from build123d import *

# Parameters (mm, degrees)
SKETCH1_W           = 3
SKETCH1_H           = 7
BOSS_EXTRUDE1_DEPTH = 3


with BuildPart() as part:
    # Sketch1 → Boss-Extrude1 (new body)
    with BuildSketch(Plane(origin=(0, 0, 0), x_dir=(0, 0, -1), z_dir=(1, 0, 0))):
        Polygon((0, 50), (-10, 50), (-10, 0), (137.373870973, 0), (137.373870973, 3.192533317), (8.7714132, 50), align=None)
        Polygon((10.422986638, 46.206343112), (9.396926208, 43.387265249), (21.612930278, 38.941003386), (22.638990708, 41.760081248), align=None, mode=Mode.SUBTRACT)
        Polygon((34.854994778, 37.313819385), (33.828934348, 34.494741523), (46.044938419, 30.04847966), (47.070998848, 32.867557522), align=None, mode=Mode.SUBTRACT)
        Polygon((119.34096284, 3.37090848), (120.36702327, 6.189986343), (108.1510192, 10.636248206), (107.12495877, 7.817170343), align=None, mode=Mode.SUBTRACT)
        Polygon((95.935015129, 15.082510069), (94.908954699, 12.263432207), (82.692950629, 16.70969407), (83.719011059, 19.528771932), align=None, mode=Mode.SUBTRACT)
        Polygon((59.287002919, 28.421295659), (58.260942489, 25.602217796), (70.476946559, 21.155955933), (71.503006989, 23.975033796), align=None, mode=Mode.SUBTRACT)
        with Locations((-5.5, 38.5)):
            Rectangle(SKETCH1_W, SKETCH1_H, mode=Mode.SUBTRACT)
        with Locations((-5.5, 24.5)):
            Rectangle(SKETCH1_W, SKETCH1_H, mode=Mode.SUBTRACT)
        with Locations((-5.5, 10.5)):
            Rectangle(SKETCH1_W, SKETCH1_H, mode=Mode.SUBTRACT)
    extrude(amount=BOSS_EXTRUDE1_DEPTH)


solid = part.part
Can you work these out from the model? Positions are in its coordinate system, mm. A direction names the side the tool comes from. Coordinates: 2 decimals unless noted, no trailing zeros. Order: outer loops, then holes, each group sorted by start corner. A loop starts at its lowest first (then second) coordinate and runs counter-clockwise, first axis right, second up. Notation, with made-up numbers: (81, 77.25) - (108, 77.25) arc R34 cw to (108, 113.25) - close; hole circle Ø7 at (-31.5, 89). An arc over 180 degrees is marked (long way). Answer as a JSON object with one key per item and string values. Group by question number.
Q1. Imagine slicing it at C-C (x = 1.6). Give the number of separate pieces and of enclosed holes in the cut face, and give its area (3 significant figures).
Q2. We'd pull the mould along Z, two halves only. Please class faces 3 (the face through (1.479, 9.246, -107.645)), 4 (the face through (1, 2, -137.374)), 5 (the face through (1, 25, 10)), 6 (the face through (0, 20, -30)): +Z half, -Z half, draft (parallel to the pull), parting line (faces both ways), or undercut.
Q3. Will this pin go through, and if not, where does the flat tip stop? P1, Ø1.5, axis at y = 19.5, z = -79.5, coming from the -X side.
Q4. Imagine slicing it at A-A (z = -61.5). Please give me the cut outline in (x, y).
Q5. I need wall thicknesses on line 1 (Y direction, x = 0.6, z = -114.5); line 2 (Y direction, x = 0.7, z = -21); line 3 (Y direction, x = 2.8, z = -57.5). Which ranges of each line are inside material? Lowest first, please. Write a range as from..to.
Q6. Imagine slicing it at D-D (z = -115). Please give me the cut outline in (x, y).
Q7. On a 3-axis mill with a long thin cutter (end or side, diameter ignored), from which of +Z, -Z, +X, -X, +Y, -Y can I reach the whole of each face in a straight line? I mean faces 1 (the face through (1, 21, 6)), 2 (the face through (1.48, 26.27, -73.97)). Say none if no direction works.
Q8. Imagine slicing it at B-B (y = 40.5). Please give me the cut outline in (x, z), and give its area (3 significant figures).
Determined:
{
 "1": {"separate pieces": "1", "enclosed holes": "8", "area": "4,100 mm2"},
 "2": {"face 3": "undercut", "face 4": "-Z half", "face 5": "+Z half", "face 6": "draft"},
 "3": {"P1": "stops at x = 0"},
 "4": {"outline": "(0, 0) - (3, 0) - (3, 24.42) - (0, 24.42) - close; (0, 27.62) - (3, 27.62) - (3, 30.81) - (0, 30.81) - close"},
 "5": {"line 1": "y = 0..5.13, 8.33..11.52", "line 2": "y = 0..39.16, 42.36..45.55", "line 3": "y = 0..32.26"},
 "6": {"outline": "(0, 0) - (3, 0) - (3, 4.95) - (0, 4.95) - close; (0, 8.14) - (3, 8.14) - (3, 11.34) - (0, 11.34) - close"},
 "7": {"face 1": "+X, -X", "face 2": "-Z, +X, -X, +Y"},
 "8": {"outline": "(0, -34.87) - (3, -34.87) - (3, -22.18) - (0, -22.18) - close; (0, -17.33) - (3, -17.33) - (3, 4) - (0, 4) - close; (0, 7) - (3, 7) - (3, 10) - (0, 10) - close", "area": "111 mm2"}
}
